Print and shaded views of the part. All mm, measured from the part's lowest x, y and z. A direction names the side the tool comes from. Coordinates: 2 decimals unless noted, no trailing zeros. Loops run counter-clockwise (first coordinate to the right, second up) from the corner with the lowest first, then second, coordinate; pieces in that order, holes last. Notation, with made-up numbers: M 31.25,85 L 57.25,85 A17 cw 57.25,108 Z; hole C 9,5 d9. An arc over 180 degrees is marked long. Use a Markdown table: item, result. Add a question column.
1) Band-saw the part on B-B (y = 4). List the corners of the cut face in (x, z).
2) Pull direction X, two halves, no side cores. Call the marked faces 1, 2, 3 and 4: released by +X, released by -X, zero draft, split by the parting line, or undercut.
3) Pin check, flat tip, straight feed: pin 1 Ø1 at (y, z) = (1, 1) entering from -X. Stop position of the tip, or through.
4) Wall check: probe 1 along Y at (x, z) = (4, 1.6); probe 2 along Y at (x, z) = (4, 0.25); probe 3 along X at (y, z) = (4.5, 0.6). Give the ranges that are in metal, low to high. Write a range as from..to.
5) Band-saw the part on D-D (z = 0.8). List the corners of the cut face in (x, y).
6) Band-saw the part on C-C (x = 1.75). List the corners of the cut face in (y, z), plus the area to 3 significant figures.
7) Tool access for the marked faces 5 and 6: list every direction of +Z, -Z, +X, -X, +Y, -Y with a clear straight run to the whole face (end or side of a thin tool).
8) Band-saw the part on A-A (x = 4). List the corners of the cut face in (y, z).
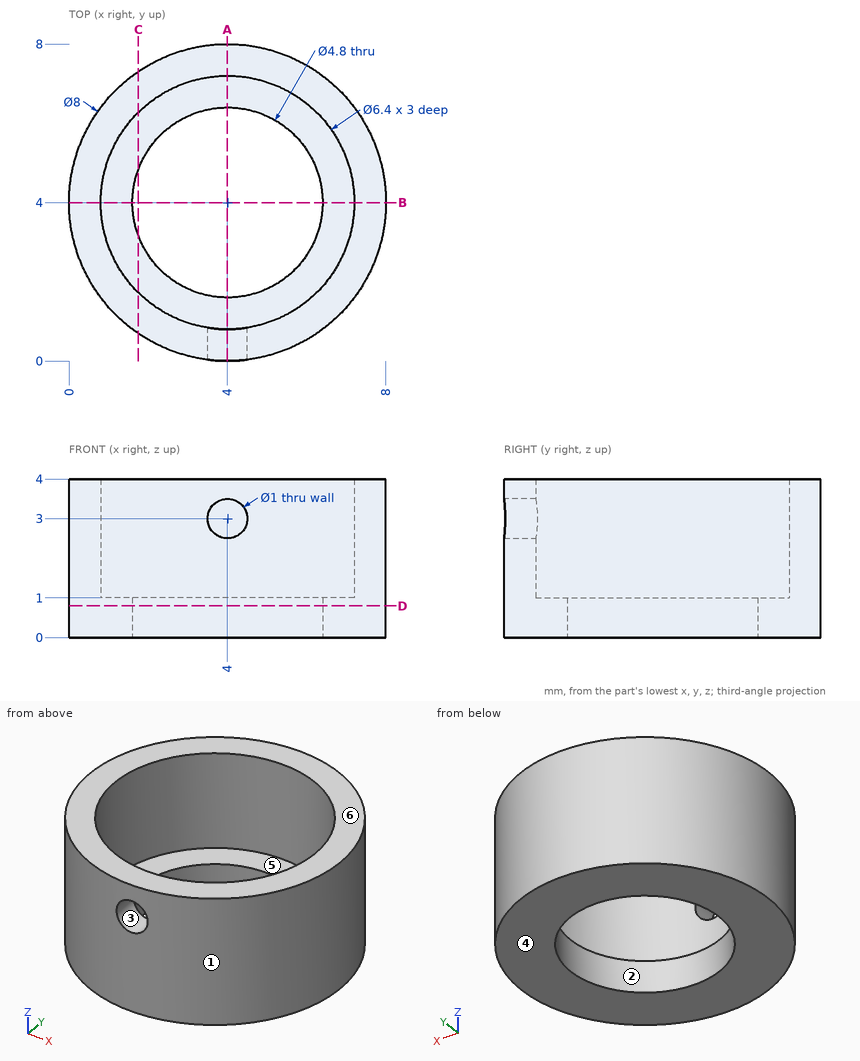
Entries:
| question | item | result |
|---|---|---|
| 1 | outline | M 0,0 L 1.6,0 L 1.6,1 L 0.8,1 L 0.8,4 L 0,4 Z; M 6.4,0 L 8,0 L 8,4 L 7.2,4 L 7.2,1 L 6.4,1 Z |
| 2 | face 1 | split by the parting line |
| 2 | face 2 | undercut |
| 2 | face 3 | undercut |
| 2 | face 4 | zero draft |
| 3 | pin 1 | x = 0.88 |
| 4 | probe 1 | 0..0.8, 7.2..8 |
| 4 | probe 2 | 0..1.6, 6.4..8 |
| 4 | probe 3 | 0.03..1.65, 6.35..7.97 |
| 5 | outline | C 4,4 d8; hole C 4,4 d4.8 |
| 6 | outline | M 0.69,0 L 3.16,0 L 3.16,1 L 1.72,1 L 1.72,4 L 0.69,4 Z; M 4.84,0 L 7.31,0 L 7.31,4 L 6.28,4 L 6.28,1 L 4.84,1 Z |
| 6 | area | 11.1 mm2 |
| 7 | face 5 | +Z |
| 7 | face 6 | +Z, +X, -X, +Y, -Y |
| 8 | outline | M 0,0 L 1.6,0 L 1.6,1 L 0.8,1 L 0.8,2.5 L 0,2.5 Z; M 0,3.5 L 0.8,3.5 L 0.8,4 L 0,4 Z; M 6.4,0 L 8,0 L 8,4 L 7.2,4 L 7.2,1 L 6.4,1 Z |
